The model under review builds one solid part; all positions refer to its coordinate system, in mm. A direction names the side the tool comes from. Give positions to 0.01 mm unless a question says otherwise; leave off trailing zeros. Write each loop counter-clockwise with the first axis right and the second up, starting at its lowest first coordinate (ties: lowest second). Pieces come first, ordered by that corner, then holes. Notation, with made-up numbers: (-38, 73) -> (21, 73) arc R13 cw to (21, 82) -> close; hole circle Ø9 at (56.5, -38.75). An arc over 180 degrees is marked (long way). Use CSV: the item, a comma, the result in double quotes.
```python
from build123d import *

# Parameters (mm, degrees)
ESQUISSE1_W        = 12
ESQUISSE1_H        = 10
BOSS_EXTRU_1_DEPTH = 9
BOSS_EXTRU_2_DEPTH = 10
BOSS_EXTRU_3_DEPTH = 16
BOSS_EXTRU_4_DEPTH = 6


with BuildPart() as part:
    # Esquisse1 → Boss.-Extru.1 (new body)
    with BuildSketch(Plane.XY):
        Rectangle(ESQUISSE1_W, ESQUISSE1_H)
    extrude(amount=BOSS_EXTRU_1_DEPTH)

    # Esquisse2 → Boss.-Extru.2 (add)
    with BuildSketch(Plane.XY.offset(9)):
        with BuildLine():
            Line((-1, 1.118033989), (1, 1.118033989))
            ThreePointArc((1, 1.118033989), (0, -1.5), (-1, 1.118033989))
        make_face()
    extrude(amount=BOSS_EXTRU_2_DEPTH)

    # Esquisse3 → Boss.-Extru.3 (add)
    with BuildSketch(Plane(origin=(0, 0, 0), x_dir=(-1, 0, 0), z_dir=(0, 0, -1))):
        with BuildLine():
            Line((-3.31662479, 5), (3.31662479, 5))
            ThreePointArc((3.31662479, 5), (6, 0), (3.31662479, -5))
            Line((3.31662479, -5), (-3.31662479, -5))
            ThreePointArc((-3.31662479, -5), (-6, 0), (-3.31662479, 5))
        make_face()
    extrude(amount=BOSS_EXTRU_3_DEPTH)

    # Esquisse4 → Boss.-Extru.4 (add)
    with BuildSketch(Plane(origin=(0, 0, -16), x_dir=(-1, 0, 0), z_dir=(0, 0, -1))):
        with BuildLine():
            Line((-3.31662479, -5), (3.31662479, -5))
            ThreePointArc((3.31662479, -5), (5.286764074, -2.837274331), (6, 0))
            Line((6, 0), (6, 13))
            Line((6, 13), (-6, 13))
            Line((-6, 13), (-6, 0))
            ThreePointArc((-6, 0), (-5.286764074, -2.837274331), (-3.31662479, -5))
        make_face()
    extrude(amount=BOSS_EXTRU_4_DEPTH)


solid = part.part
```
Q1. Consider section A-A (x = 2.75). Write out the cut boundary in (y, z).
Derived:
outline,"(-5, -22) -> (13, -22) -> (13, -16) -> (5, -16) -> (5, 9) -> (-5, 9) -> close"
Q2. Insertion check: pin 1 (1 mm diameter, centred on y = 6, z = -9, fed in from +X); pin 2 (0.6 mm diameter, centred on x = -0.5, z = 12.5, fed in from +Y); pin 3 (2 mm diameter, centred on y = 2, z = -1.5, fed in from +X); pin 4 (3 mm diameter, centred on x = 4, z = -8, fed in from +Y). Each pin has a flat end and moves straight along its axis. Give the tip position at first contact, or say it passes through.
Derived:
pin 1,"passes through"
pin 2,"stops at y = 1.12"
pin 3,"stops at x = 5.92"
pin 4,"stops at y = 5"
Q3. The part is to be moulded in two halves that separate along Z. For faces 5 (the flat face through (1.2, 1.2, 9)), 6 (the flat face through (-5, 4, 0)), 7 (the flat face through (6, 7, -19)), 8 (the flat face through (5, 4, 0)), say which applies: pulls with the +Z half, pulls with the -Z half, needs draft (parallel to the pull), parting line crosses it, or undercut.
Derived:
face 5,"pulls with the +Z half"
face 6,"undercut"
face 7,"needs draft"
face 8,"undercut"
Q4. Consider section B-B (y = -2.75). Write out the cut boundary in (x, z).
Derived:
outline,"(-6, 0) -> (-5.33, 0) -> (-5.33, -22) -> (5.33, -22) -> (5.33, 0) -> (6, 0) -> (6, 9) -> (-6, 9) -> close"
Q5. Machinability: for faces 1 (the flat face through (-5, -4, 0)), 2 (the cylindrical face through (0.05, -1.5, 13.93)), 3 (the flat face through (0, 5, -1)), 4 (the flat face through (5, -4, 0)), which of the approach directions +Z, -Z, +X, -X, +Y, -Y give a long, thin tool a straight path to every point of the face, cutting with its end or side? Answer none if there is none.
Derived:
face 1,"-Z, -X, -Y"
face 2,"+Z"
face 3,"+Z, +X, -X, +Y"
face 4,"-Z, +X, -Y"
Q6. Consider section D-D (x = 0). Write out the cut boundary in (y, z), then the cut area to 3 significant figures.
Derived:
outline,"(-5, -22) -> (13, -22) -> (13, -16) -> (5, -16) -> (5, 9) -> (1.12, 9) -> (1.12, 19) -> (-1.5, 19) -> (-1.5, 9) -> (-5, 9) -> close"
area,"384 mm2"
Q7. Consider section C-C (z = -1). Write out the cut boundary in (x, y), then the cut area to 3 significant figures.
Derived:
outline,"(-3.32, -5) -> (3.32, -5) arc R6 ccw to (3.32, 5) -> (-3.32, 5) arc R6 ccw to start"
area,"104 mm2"
Q8. To check wall thickness, follow probe 1 along Z at (x, y) = (5, 3.5); probe 2 along Z at (x, y) = (-0.5, 11.75); probe 3 along Z at (x, y) = (-4.25, -0.5). State the ranges of each line that lie inside material, in increasing order.
Derived:
probe 1,"z = -22 to -16, 0 to 9"
probe 2,"z = -22 to -16"
probe 3,"z = -22 to 9"
